The model under review builds one solid part; all positions refer to its coordinate system, in mm. A direction names the side the tool comes from. Coordinates: 2 decimals unless noted, no trailing zeros. Write each loop counter-clockwise with the first axis right and the second up, starting at its lowest first coordinate (ties: lowest second). Pieces come first, ordered by that corner, then holes. Notation, with made-up numbers: M 81.25,-4 L 90.25,-4 A30 cw 90.25,23 Z; hole C 57,62 d8. An arc over 180 degrees is marked long. Answer as a JSON object with one key per item and string values.
```python
from build123d import *

# Parameters (mm, degrees)
F0_W     = 133.2367658615
F0_H     = 109.6848323941
F1_DEPTH = 87.122
F3_DEPTH = 18.542
F4_DEPTH = 140.208
F6_DEPTH = 25.4
F7_R     = 9.8377805887
F8_DEPTH = 150.876
F7_R_2   = 11.4915117279
F9_DEPTH = 154.432


with BuildPart() as f1:
    # F0 (on Top) → F1 (new body)
    with BuildSketch(Plane.XY):
        with Locations((-3.2847598195, 4.5694448054)):
            Rectangle(F0_W, F0_H)
    extrude(amount=F1_DEPTH)

    # F2 (on face) → F3 (join)
    with BuildSketch(Plane.XZ.offset(50.2729713917)):
        with BuildLine():
            Line((-20.3312505037, 87.122), (-33.694114536, 87.122))
            ThreePointArc((-33.694114536, 87.122), (-1.149084419, 58.9054568652), (31.395945698, 87.122))
            Line((31.395945698, 87.122), (21.0505016148, 87.122))
            ThreePointArc((21.0505016148, 87.122), (0.3596255556, 70.4522292625), (-20.3312505037, 87.122))
        make_face()
    extrude(amount=F3_DEPTH)

    # F4 (cut): a face of the model
    f4_faces = [f1.faces().sort_by_distance(p)[0] for p in [
        (0.3596255556, -50.2729713917, 80.1609892237),
    ]]
    extrude(f4_faces, amount=-F4_DEPTH, mode=Mode.SUBTRACT)

    # F5 (on face) → F6 (join)
    with BuildSketch(Plane(origin=(0, 59.4118610024, 0), x_dir=(-1, 0, 0), z_dir=(0, 1, 0))):
        with BuildLine():
            Line((-21.0505016148, 87.122), (-32.8814908862, 87.122))
            ThreePointArc((-32.8814908862, 87.122), (0.5957707763, 58.2968596354), (34.0730324388, 87.122))
            Line((34.0730324388, 87.122), (20.3312505037, 87.122))
            ThreePointArc((20.3312505037, 87.122), (-0.3596255556, 70.4522292625), (-21.0505016148, 87.122))
        make_face()
    extrude(amount=F6_DEPTH)

    # F7 (on face) → F8 (cut)
    with BuildSketch(Plane.XY.offset(87.122)):
        with Locations((-50.3509901464, 3.0695819296)):
            Circle(F7_R)
    extrude(amount=-F8_DEPTH, mode=Mode.SUBTRACT)

    # F7 (on face) → F9 (cut)
    with BuildSketch(Plane.XY.offset(87.122)):
        with Locations((49.7736558318, 0)):
            Circle(F7_R_2)
    extrude(amount=-F9_DEPTH, mode=Mode.SUBTRACT)


solid = f1.part
```
(1) Add section D-D on y = 30. Give the boundary of the cut face in (x, z).
Results list:
{"outline": "M -69.9,0 L 63.33,0 L 63.33,87.12 L 21.05,87.12 A21.18 cw -20.33,87.12 L -69.9,87.12 Z"}
(2) For pin 1 Ø1.5 at (x, z) = (-50.5, 13.5) entering from +Y, flat-tipped, find the tip position at first contact; note if it passes through.
Results list:
{"pin 1": "y = 59.41"}
(3) Add section A-A on y = 6. Give the boundary of the cut face in (x, z), and give its area (3 significant figures).
Results list:
{"outline": "M -69.9,0 L -59.74,0 L -59.74,87.12 L -69.9,87.12 Z; M -40.96,0 L 39.97,0 L 39.97,87.12 L 21.05,87.12 A21.18 cw -20.33,87.12 L -40.96,87.12 Z; M 59.57,0 L 63.33,0 L 63.33,87.12 L 59.57,87.12 Z", "area": "7,750 mm²"}
(4) Draft analysis for pull direction Y (two halves, no side actions). For faces 1 (the face through (-69.903, 4, 43)), 2 (the face through (-52.484, -6.534, 44.171)), 3 (the face through (-4, -50.273, 43)), state which applies: released by +Y, released by -Y, zero draft, split by the parting line, or undercut.
Results list:
{"face 1": "zero draft", "face 2": "undercut", "face 3": "released by -Y"}
(5) Add section C-C on z = 68.5. Give the boundary of the cut face in (x, y), and give its area (3 significant figures).
Results list:
{"outline": "M -69.9,-50.27 L -24.36,-50.27 L -24.36,-68.81 L 22.06,-68.81 L 22.06,-50.27 L 63.33,-50.27 L 63.33,59.41 L 23.63,59.41 L 23.63,84.81 L -24.82,84.81 L -24.82,59.41 L -69.9,59.41 Z; hole C -50.35,3.07 d19.68; hole C 49.77,0 d22.98", "area": "16,000 mm²"}
(6) Add section B-B on x = -8. Give the boundary of the cut face in (y, z).
Results list:
{"outline": "M -68.81,59.63 L -50.27,59.63 L -50.27,0 L 59.41,0 L 59.41,59.12 L 84.81,59.12 L 84.81,72.17 L -68.81,72.17 Z"}
(7) For faces 4 (the face through (0.078, 71.934, 58.304)), 5 (the face through (-1.807, -59.414, 58.912)), 6 (the face through (63.334, 4, 43)), list the 3-axis set-ups (+Z, -Z, +X, -X, +Y, -Y) from which the entire face can be reached by the end or side of a thin tool; tool diameter is ignored.
Results list:
{"face 4": "-Z, +Y", "face 5": "-Z, -Y", "face 6": "+Z, -Z, +X, +Y, -Y"}
(8) Wall thickness on line 1 along X through (y, z) = (-2, 57); line 2 along Y through (x, z) = (34, 83); line 3 along X through (y, z) = (-35, 77.5): over which ranges is each line inside the solid? List them lowest first. Write a range as from..to.
Results list:
{"line 1": "-69.9..-58.78, -41.92..38.46, 61.09..63.33", "line 2": "-50.27..59.41", "line 3": "-69.9..-15.41, 16.13..63.33"}
